Geometry: final body of the model. Coordinates: model frame, mm. A direction names the side the tool comes from. Round coordinates to 2 decimals unless told otherwise and drop trailing zeros. Order: outer loops, then holes, each group sorted by start corner. A loop starts at its lowest first (then second) coordinate and runs counter-clockwise, first axis right, second up. Notation, with made-up numbers: M 58.25,-32.5 L 97.25,-32.5 A17 cw 97.25,-8.5 Z; hole C -31,52.5 d2. An arc over 180 degrees is marked long. Return JSON: item names as keys, results as strings. Group by question number.
Q1. Cut plane B-B on x = -12.5. Output: boundary loops of the cut face in (y, z), and give its area (3 significant figures).
Q2. Ray query, probe 1 along Y at (x, z) = (0, 2.5); probe 2 along Y at (x, z) = (-94, 2.25); probe 3 along X at (y, z) = (1, 2.5). Return the intervals inside material, ascending.
Q3. Access query for faces 5 (the face through (-65, 51.359, 3)), 6 (the face through (-129.56, 0.16, 3.04)). Directions: +Z, -Z, +X, -X, +Y, -Y. A direction counts if a zero-diameter tool reaches every point of the face in a straight line with its end or side. Return the directions, or none.
Q4. Mould query, pull axis X, two halves, no side actions, for faces 1 (the face through (2.192, -4.214, 3.043)), 2 (the face through (-153.3, 0, 3)), 3 (the face through (24.5, 0, 3)), 4 (the face through (-64, -51.359, 3)). Classes: released by +X, released by -X, zero draft, split by the parting line, or undercut.
Q5. Cut plane A-A on y = 12.5. Output: boundary loops of the cut face in (x, z), and give its area (3 significant figures).
Q6. Cut plane C-C on x = -66. Output: boundary loops of the cut face in (y, z).
Q7. Cut plane D-D on z = 1.75. Count the separate pieces of the cut face and the enclosed holes in it, and give its area (3 significant figures).
Q8. Contact query for flat-ended pins moving along their axis: pin 1 (3 mm diameter, centred on x = 0, y = -12.5, fed in from +Z); pin 2 (3 mm diameter, centred on y = 35, z = 1.5, fed in from -X). Output: stop coordinate, or through.
```python
from build123d import *

# Parameters (mm, degrees)
SKETCH1_R           = 1.65
SKETCH1_R_2         = 4.75
BOSS_EXTRUDE1_DEPTH = 6.1722
CUT_EXTRUDE1_DEPTH  = 162.792188904


with BuildPart() as part:
    # Sketch1 → Boss-Extrude1 (new body)
    with BuildSketch(Plane.XY):
        with BuildLine():
            Line((-0.9, -51.3588), (-127.9, -51.3588))
            ThreePointArc((-127.9, -51.3588), (-145.860512242, -43.919312242), (-153.3, -25.9588))
            Line((-153.3, -25.9588), (-153.3, 25.9588))
            ThreePointArc((-153.3, 25.9588), (-145.860512242, 43.919312242), (-127.9, 51.3588))
            Line((-127.9, 51.3588), (-0.9, 51.3588))
            ThreePointArc((-0.9, 51.3588), (17.060512242, 43.919312242), (24.5, 25.9588))
            Line((24.5, 25.9588), (24.5, -25.9588))
            ThreePointArc((24.5, -25.9588), (17.060512242, -43.919312242), (-0.9, -51.3588))
        make_face()
        with Locations((12.5, 0)):
            Circle(SKETCH1_R, mode=Mode.SUBTRACT)
        with Locations((0, -12.5)):
            Circle(SKETCH1_R, mode=Mode.SUBTRACT)
        with Locations((-12.5, 0)):
            Circle(SKETCH1_R, mode=Mode.SUBTRACT)
        with Locations((0, 12.5)):
            Circle(SKETCH1_R, mode=Mode.SUBTRACT)
        Circle(SKETCH1_R_2, mode=Mode.SUBTRACT)
    extrude(amount=BOSS_EXTRUDE1_DEPTH)

    # Sketch2 → Cut-Extrude1 (cut, through all)
    with BuildSketch(Plane(origin=(0, 0, 0), x_dir=(-1, 0, 0), z_dir=(0, 0, -1))):
        with BuildLine():
            Line((44.019348423, 29.52115), (107.591551577, 29.52115))
            ThreePointArc((107.591551577, 29.52115), (112.633451577, 24.47925), (107.591551577, 19.43735))
            Line((107.591551577, 19.43735), (44.019348423, 19.43735))
            ThreePointArc((44.019348423, 19.43735), (38.977448423, 24.47925), (44.019348423, 29.52115))
        make_face()
        with BuildLine():
            Line((44.019348423, -19.43735), (107.591551577, -19.43735))
            ThreePointArc((107.591551577, -19.43735), (112.633451577, -24.47925), (107.591551577, -29.52115))
            Line((107.591551577, -29.52115), (44.019348423, -29.52115))
            ThreePointArc((44.019348423, -29.52115), (38.977448423, -24.47925), (44.019348423, -19.43735))
        make_face()
        with BuildLine():
            Line((35.080546846, 7.4422), (122.118353154, 7.4422))
            ThreePointArc((122.118353154, 7.4422), (129.560553154, 0), (122.118353154, -7.4422))
            Line((122.118353154, -7.4422), (35.080546846, -7.4422))
            ThreePointArc((35.080546846, -7.4422), (27.638346846, 0), (35.080546846, 7.4422))
        make_face()
    extrude(amount=-CUT_EXTRUDE1_DEPTH, mode=Mode.SUBTRACT)


solid = part.part
```
Result sheet:
{
 "1": {"outline": "M -51.36,0 L -1.65,0 L -1.65,6.17 L -51.36,6.17 Z; M 1.65,0 L 51.36,0 L 51.36,6.17 L 1.65,6.17 Z", "area": "614 mm²"},
 "2": {"probe 1": "y = -51.34 to -14.15, -10.85 to -4.75, 4.75 to 10.85, 14.15 to 51.34", "probe 2": "y = -51.36 to -29.52, -19.44 to -7.44, 7.44 to 19.44, 29.52 to 51.36", "probe 3": "x = -153.3 to -129.49, -27.71 to -13.81, -11.19 to -4.64, 4.64 to 11.19, 13.81 to 24.5"},
 "3": {"face 5": "+Z, -Z, +X, -X, +Y", "face 6": "+Z, -Z"},
 "4": {"face 1": "undercut", "face 2": "released by -X", "face 3": "released by +X", "face 4": "zero draft"},
 "5": {"outline": "M -153.3,0 L -1.65,0 L -1.65,6.17 L -153.3,6.17 Z; M 1.65,0 L 24.5,0 L 24.5,6.17 L 1.65,6.17 Z", "area": "1,080 mm²"},
 "6": {"outline": "M -51.36,0 L -29.52,0 L -29.52,6.17 L -51.36,6.17 Z; M -19.44,0 L -7.44,0 L -7.44,6.17 L -19.44,6.17 Z; M 7.44,0 L 19.44,0 L 19.44,6.17 L 7.44,6.17 Z; M 29.52,0 L 51.36,0 L 51.36,6.17 L 29.52,6.17 Z"},
 "7": {"separate pieces": "1", "enclosed holes": "8", "area": "14,700 mm²"},
 "8": {"pin 1": "passes through", "pin 2": "stops at x = -152.15"}
}
